Solid Edge part; units mm, degrees
sketch "Sketch1" plane through (0, 0, 0) normal (0, 0, 1) x (1, 0, 0)
  circle A0 centre (-52.9419, 44.7949) radius 50
revolve "RevolvedProtrusion1" add sketch "Sketch1" angle 360 about axis through (17.0581, 73.3637, 0) along (0, -1, 0)
sketch "Sketch2" plane through (0, -147.6255, 0) normal (0, -1, 0) x (1, 0, 0)
  line L0 (17.0581, 0) -> (-138.6485, -80.2172)
  line L1 (-138.6485, -80.2172) -> (0, -167.5212)
  line L2 (0, -167.5212) -> (171.0814, -99.0457)
  line L3 (171.0814, -99.0457) -> (17.0581, 0)
extrude "Cutout1" cut sketch "Sketch2" against normal through all
sketch "Sketch3" plane through (0, 0, 170.0341) normal (0, 0, 1) x (1, 0, 0)
  line L0 (12.0581, 39.7949) -> (22.0581, 39.7949)
  line L1 (22.0581, 39.7949) -> (22.0581, 49.7949)
  line L2 (22.0581, 49.7949) -> (12.0581, 49.7949)
  line L3 (12.0581, 49.7949) -> (12.0581, 39.7949)
  dimension "D1" = 22.0581
  dimension "D2" = 12.0581
extrude "ExtrudedCutout_5" cut sketch "Sketch3" against normal blind 100
sketch "Sketch4" plane through (0, 44.7949, 0) normal (0, -1, 0) x (1, 0, 0)
  line L0 (-114.5124, -54.9573) -> (-114.5124, -59.5106)
  line L1 (-114.5124, -59.5106) -> (-108.2396, -59.5106)
  line L2 (-108.2396, -59.5106) -> (-108.2396, -54.9573)
  line L3 (-108.2396, -54.9573) -> (-114.5124, -54.9573)
  circle A0 centre (-111.5124, -57.3579) radius 1
  line L4 (-89.6175, -54.9573) -> (-114.6175, -54.9573)
  line L5 (-114.6175, -54.9573) -> (-114.6175, -50.3942)
  line L6 (-114.6175, -50.3942) -> (-87.7233, -50.3942)
  line L7 (-87.7233, -50.3942) -> (-89.6175, -54.9573)
  dimension "D1" = 89.6175
extrude "ExtrudedProtrusion_1" add sketch "Sketch4" against normal blind 4
For this review, take the finished solid that the model builds, in its own axes (mm). A direction names the side the tool comes from. Give positions to 0.01 mm unless a question says otherwise; leave off trailing zeros. Order: outer loops, then holes, each group sorted by start corner. A loop starts at its lowest first (then second) coordinate and runs counter-clockwise, first axis right, second up. Notation, with made-up numbers: M 69,8.5 L 122,8.5 A10 cw 122,14.5 Z; hole C 72.25,2.5 d9. An arc over 180 degrees is marked long. Answer in a Markdown table with one row per item. Add a question column.
(1) Consider section A-A on y = 16.5. State the section outline as (x, z) points.
(2) Consider section B-B on y = 68.5. State the section outline as (x, z) points.
(3) For faces 5 (the face through (12.058, 45, 95)), 6 (the face through (76.527, 44.095, -38.242)), list the 3-axis set-ups (+Z, -Z, +X, -X, +Y, -Y) from which the entire face can be reached by the end or side of a thin tool; tool diameter is ignored.
(4) For pin 1 (5 mm diameter, centred on x = -27, y = 36, fed in from -Z); pin 2 (1.2 mm diameter, centred on x = -112.5, y = 46.5, fed in from -Z); pin 3 (5 mm diameter, centred on y = 45.5, z = 107, fed in from +X), all flat-tipped, find the tip position at first contact; note any pin that passes through.
(5) Wall thickness on probe 1 along Y at (x, z) = (-46, -27.5); probe 2 along X at (y, z) = (49, -36); probe 3 along X at (y, z) = (66, -49): over which ranges is each line inside the solid? List them lowest first. Write a range as [from, to].
(6) Mouldability with a two-part tool opening along Y and no side actions: class faces 1 (the face through (-105, 48.795, -54)), 2 (the face through (17, 45, 70.034)), 3 (the face through (22.058, 45, 95)), 4 (the face through (-105, 44.795, -54)) as +Y half, -Y half, draft (parallel to the pull), parting line (faces both ways), or undercut.
Evaluation:
| question | item | result |
|---|---|---|
| 1 | outline | M -81.82,-50.94 L -8.52,-13.18 A28.78 cw long 41.26,-15.56 L 110.61,-60.16 A111.22 ccw long Z |
| 2 | outline | M -84.3,-52.22 L -6.03,-11.9 A25.98 cw long 38.91,-14.05 L 112.96,-61.67 A114.02 ccw long Z |
| 3 | face 5 | +Z |
| 3 | face 6 | -Z, +Y, -Y |
| 4 | pin 1 | stops at z = -23.99 |
| 4 | pin 2 | stops at z = -59.51 |
| 4 | pin 3 | stops at x = 76.04 |
| 5 | probe 1 | y = [-5.19, 94.78] |
| 5 | probe 2 | x = [-97.23, -52.82], [73.04, 131.35] |
| 5 | probe 3 | x = [-87.29, -78.05], [93.26, 121.41] |
| 6 | face 1 | +Y half |
| 6 | face 2 | undercut |
| 6 | face 3 | undercut |
| 6 | face 4 | -Y half |
